Print and shaded views of the part. All mm, measured from the part's lowest x, y and z. A direction names the side the tool comes from. Round coordinates to 2 decimals unless told otherwise and drop trailing zeros. Write each loop counter-clockwise with the first axis right and the second up, starting at its lowest first coordinate (ties: lowest second). Pieces come first, ordered by that corner, then holes. Notation, with made-up numbers: (-17, -23) - (-9, -23) arc R38 ccw to (-9, 15) - close; hole circle Ø3 at (45, 33.25). An arc over 180 degrees is marked (long way). One line per item, written item: value.
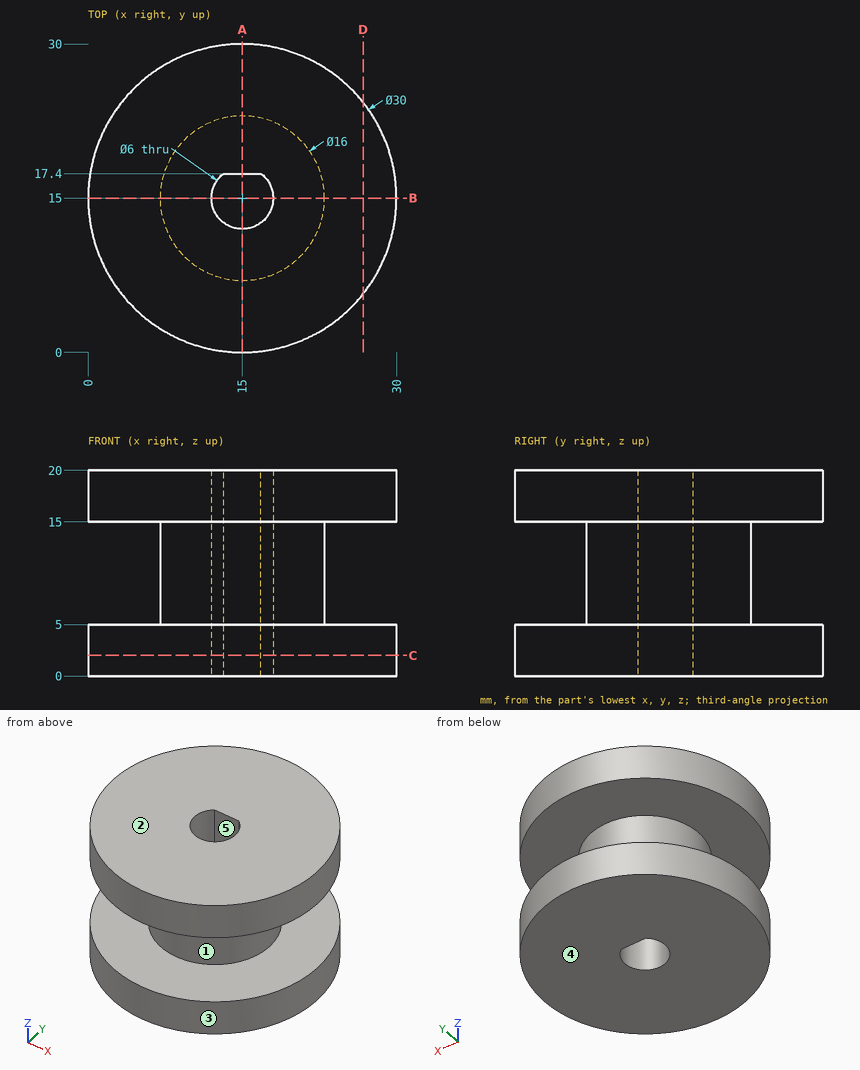
1. Band-saw the part on B-B on y = 15. Write the cut outline in (x, z).
Report:
outline: (0, 0) - (12, 0) - (12, 20) - (0, 20) - (0, 15) - (7, 15) - (7, 5) - (0, 5) - close; (18, 0) - (30, 0) - (30, 5) - (23, 5) - (23, 15) - (30, 15) - (30, 20) - (18, 20) - close
2. Band-saw the part on D-D on x = 26.75. Write the cut outline in (y, z).
Report:
outline: (5.68, 0) - (24.32, 0) - (24.32, 5) - (5.68, 5) - close; (5.68, 15) - (24.32, 15) - (24.32, 20) - (5.68, 20) - close
3. Mould opens along Y. For the marked faces 3, 4 and 5 say: released by +Y, released by -Y, zero draft, split by the parting line, or undercut.
Report:
face 3: split by the parting line
face 4: zero draft
face 5: undercut
4. Wall check: probe 1 along Y at (x, z) = (15, 10.25); probe 2 along Z at (x, y) = (19.5, 22.25); probe 3 along Y at (x, z) = (17.5, 5.5). Give the ranges that are in metal, low to high. Write a range as [from, to].
Report:
probe 1: [7, 12], [17.4, 23]
probe 2: [0, 5], [15, 20]
probe 3: [7.4, 13.34], [16.66, 22.6]
5. Drop flat-ended pins along their axis: pin 1 (1.5 mm diameter, centred on x = 16.5, z = 7, fed in from -Y); pin 2 (8 mm diameter, centred on y = 20, z = 13, fed in from +X); pin 3 (8 mm diameter, centred on x = 10, z = 13.5, fed in from +Y); pin 4 (3.5 mm diameter, centred on x = 15, y = 15, fed in from -Z). Give the stop position or say it passes through.
Report:
pin 1: y = 7.04
pin 2: x = 29.92
pin 3: y = 29.94
pin 4: through
6. Band-saw the part on A-A on x = 15. Write the cut outline in (y, z), plus the area to 3 significant figures.
Report:
outline: (0, 0) - (12, 0) - (12, 20) - (0, 20) - (0, 15) - (7, 15) - (7, 5) - (0, 5) - close; (17.4, 0) - (30, 0) - (30, 5) - (23, 5) - (23, 15) - (30, 15) - (30, 20) - (17.4, 20) - close
area: 352 mm²
7. Tool access for the marked faces 1 and 2: list every direction of +Z, -Z, +X, -X, +Y, -Y with a clear straight run to the whole face (end or side of a thin tool).
Report:
face 1: none
face 2: +Z, +X, -X, +Y, -Y
8. Band-saw the part on C-C on z = 2. Write the cut outline in (x, y), plus the area to 3 significant figures.
Report:
outline: circle Ø30 at (15, 15); hole (13.2, 17.4) arc R3 ccw (long way) to (16.8, 17.4) - close
area: 680 mm²
